Geometry check sheet. Reference: the model listing, model coordinates, mm. Face numbers are marked on the shaded views. Give positions to 0.01 mm unless a question says otherwise; leave off trailing zeros. Loops run counter-clockwise (first coordinate to the right, second up) from the corner with the lowest first, then second, coordinate; pieces in that order, holes last. Notation, with made-up numbers: (-9, -33) -> (10, -33) arc R27 cw to (10, 3) -> close; hole circle Ø2 at (25, -13). An arc over 180 degrees is marked (long way). Answer as a JSON object with one key per item and string values.
from build123d import *

# Parameters (mm, degrees)
F0_R     = 8.201166
F1_DEPTH = 25.4
F2_SIZE  = 5.08


with BuildPart() as f1:
    # F0 (on Front) → F1 (new body)
    with BuildSketch(Plane.XZ):
        Polygon((25.464479, 20.581946), (-20.489236, 20.581946), (-20.489236, -20.025678), (54.607056, -20.025678), (54.607056, 0), align=None)
        Circle(F0_R, mode=Mode.SUBTRACT)
    extrude(amount=F1_DEPTH)

    # F2
    f2_edges = [f1.edges().sort_by_distance(p)[0] for p in [
        (25.464479, -12.7, 20.581946),
    ]]
    chamfer(f2_edges, length=F2_SIZE)


solid = f1.part
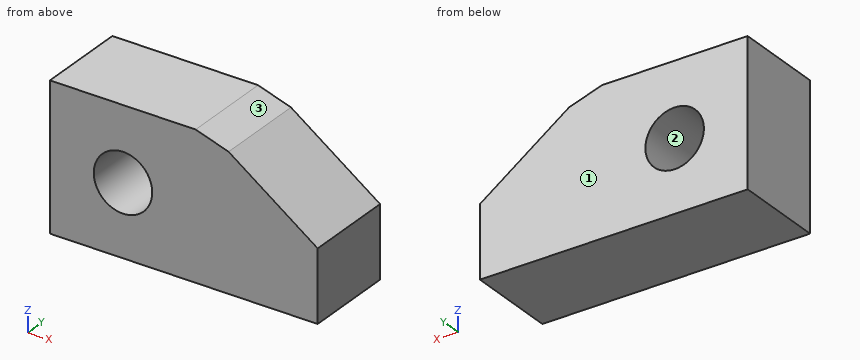
1) Depth check by flat-ended pin: P1, Ø6, axis at x = -3, z = 2.5, coming from the +Y side; P2, Ø6, axis at y = -12.5, z = 15, coming from the +X side. Enter the tip coordinate at first touch or a pass-through.
Geometry check:
{"P1": "passes through", "P2": "stops at x = 37.62"}
2) Section check D-D on x = 34. Record the cut outline in (y, z), plus the area to 3 significant figures.
Geometry check:
{"outline": "(-25.4, -20.03) -> (0, -20.03) -> (0, 14.55) -> (-25.4, 14.55) -> close", "area": "878 mm2"}
3) Section check C-C on y = -3.75. Record the cut outline in (x, z), plus the area to 3 significant figures.
Geometry check:
{"outline": "(-20.49, -20.03) -> (54.61, -20.03) -> (54.61, 0) -> (29.61, 17.65) -> (20.38, 20.58) -> (-20.49, 20.58) -> close; hole circle Ø16.4 at (0, 0)", "area": "2,530 mm2"}
4) Draft check along X on the marked faces 1, 2 and 3. Enter one of: pulls with the +X half, pulls with the -X half, needs draft (parallel to the pull), parting line crosses it, or undercut.
Geometry check:
{"face 1": "needs draft", "face 2": "undercut", "face 3": "pulls with the +X half"}
5) Material ranges on line 1 along Z through (x, y) = (0, -8.5); line 2 along Z through (x, y) = (-2.5, -10.75); line 3 along X through (y, z) = (-21.5, -7), recorded low to high. Write a range as from..to.
Geometry check:
{"line 1": "z = -20.03..-8.2, 8.2..20.58", "line 2": "z = -20.03..-7.81, 7.81..20.58", "line 3": "x = -20.49..-4.27, 4.27..54.61"}
6) Section check A-A on x = 0. Record the cut outline in (y, z), plus the area to 3 significant figures.
Geometry check:
{"outline": "(-25.4, -20.03) -> (0, -20.03) -> (0, -8.2) -> (-25.4, -8.2) -> close; (-25.4, 8.2) -> (0, 8.2) -> (0, 20.58) -> (-25.4, 20.58) -> close", "area": "615 mm2"}
7) Section check B-B on z = 1. Record the cut outline in (x, y), plus the area to 3 significant figures.
Geometry check:
{"outline": "(-20.49, -25.4) -> (-8.14, -25.4) -> (-8.14, 0) -> (-20.49, 0) -> close; (8.14, -25.4) -> (53.19, -25.4) -> (53.19, 0) -> (8.14, 0) -> close", "area": "1,460 mm2"}
